```python
from build123d import *

# Parameters (mm, degrees)
SKETCH1_W           = 98
SKETCH1_H           = 55
BOSS_EXTRUDE1_DEPTH = 2
SKETCH2_W           = 98
SKETCH2_H           = 55
SKETCH2_W_2         = 95
SKETCH2_H_2         = 52
BOSS_EXTRUDE2_DEPTH = 9
SKETCH3_R           = 4
SKETCH3_R_2         = 1.8
BOSS_EXTRUDE3_DEPTH = 7


with BuildPart() as part:
    # Sketch1 → Boss-Extrude1 (new body)
    with BuildSketch(Plane.XY):
        with Locations((49, -27.5)):
            Rectangle(SKETCH1_W, SKETCH1_H)
    extrude(amount=BOSS_EXTRUDE1_DEPTH)

    # Sketch2 → Boss-Extrude2 (add)
    with BuildSketch(Plane.XY.offset(2)):
        with Locations((49, -27.5)):
            Rectangle(SKETCH2_W, SKETCH2_H)
        with Locations((49, -27.5)):
            Rectangle(SKETCH2_W_2, SKETCH2_H_2, mode=Mode.SUBTRACT)
    extrude(amount=BOSS_EXTRUDE2_DEPTH)

    # Sketch3 → Boss-Extrude3 (add)
    with BuildSketch(Plane.XY.offset(2)):
        with Locations((89.5, -8.5)):
            Circle(SKETCH3_R)
        with Locations((89.5, -8.5)):
            Circle(SKETCH3_R_2, mode=Mode.SUBTRACT)
        with Locations((89.5, -48.5)):
            Circle(SKETCH3_R)
        with Locations((89.5, -48.5)):
            Circle(SKETCH3_R_2, mode=Mode.SUBTRACT)
        with Locations((6.5, -48.5)):
            Circle(SKETCH3_R)
        with Locations((6.5, -48.5)):
            Circle(SKETCH3_R_2, mode=Mode.SUBTRACT)
        with Locations((23.5, -8.5)):
            Circle(SKETCH3_R)
        with Locations((23.5, -8.5)):
            Circle(SKETCH3_R_2, mode=Mode.SUBTRACT)
    extrude(amount=BOSS_EXTRUDE3_DEPTH)


solid = part.part
```
Input: part model. Units: mm. Frame: model coordinates. A direction names the side the tool comes from. Round coordinates to 2 decimals unless told otherwise and drop trailing zeros. Loops run counter-clockwise (first coordinate to the right, second up) from the corner with the lowest first, then second, coordinate; pieces in that order, holes last. Notation, with made-up numbers: M 3,-35 L 40,-35 A16 ccw 40,-15 Z; hole C 34,29 d9. An arc over 180 degrees is marked long. Answer in a Markdown table with one row per item. Add a question column.
1. Section D-D (x = 45.5). Output: boundary loops of the cut face in (y, z), and give its area (3 significant figures).
2. Section C-C (y = -8.5). Output: boundary loops of the cut face in (x, z), and give its area (3 significant figures).
3. Mould query, pull axis Y, two halves, no side actions, for faces 3 (the face through (6.266, -46.715, 5.451)), 4 (the face through (48, 0, 5)), 5 (the face through (20.3, -10.9, 5.5)), 6 (the face through (98, -28, 5)). Classes: released by +Y, released by -Y, zero draft, split by the parting line, or undercut.
4. Contact query for flat-ended pins moving along their axis: pin 1 (5 mm diameter, centred on x = 39.5, y = -44, fed in from -Z); pin 2 (6.5 mm diameter, centred on x = 24, y = -10.5, fed in from +Z); pin 3 (1.1 mm diameter, centred on x = 6.5, y = -47.5, fed in from +Z). Output: stop coordinate, or through.
5. Ray query, probe 1 along Y at (x, z) = (6.5, 6.5); probe 2 along Y at (x, z) = (23.5, 7.5); probe 3 along Y at (x, z) = (89.5, 6). Return the intervals inside material, ascending.
6. Section B-B (x = 6.5). Output: boundary loops of the cut face in (y, z).
7. Set-up query: faces 1 (the face through (96.5, -28, 6)), 2 (the face through (48, -27, 0)). Return all of +Z, -Z, +X, -X, +Y, -Y with unobstructed straight access to the full face (end or side cutting, diameter ignored); none if empty.
8. Section A-A (z = 7.5). Give the number of separate pieces and of enclosed holes in the cut face, and give its area (3 significant figures).
Values follow:
| question | item | result |
|---|---|---|
| 1 | outline | M -55,0 L 0,0 L 0,11 L -1.5,11 L -1.5,2 L -53.5,2 L -53.5,11 L -55,11 Z |
| 1 | area | 137 mm^2 |
| 2 | outline | M 0,0 L 98,0 L 98,11 L 96.5,11 L 96.5,2 L 93.5,2 L 93.5,9 L 91.3,9 L 91.3,2 L 87.7,2 L 87.7,9 L 85.5,9 L 85.5,2 L 27.5,2 L 27.5,9 L 25.3,9 L 25.3,2 L 21.7,2 L 21.7,9 L 19.5,9 L 19.5,2 L 1.5,2 L 1.5,11 L 0,11 Z |
| 2 | area | 285 mm^2 |
| 3 | face 3 | undercut |
| 3 | face 4 | released by +Y |
| 3 | face 5 | undercut |
| 3 | face 6 | zero draft |
| 4 | pin 1 | z = 0 |
| 4 | pin 2 | z = 9 |
| 4 | pin 3 | z = 2 |
| 5 | probe 1 | -55 to -53.5, -52.5 to -50.3, -46.7 to -44.5, -1.5 to 0 |
| 5 | probe 2 | -55 to -53.5, -12.5 to -10.3, -6.7 to -4.5, -1.5 to 0 |
| 5 | probe 3 | -55 to -53.5, -52.5 to -50.3, -46.7 to -44.5, -12.5 to -10.3, -6.7 to -4.5, -1.5 to 0 |
| 6 | outline | M -55,0 L 0,0 L 0,11 L -1.5,11 L -1.5,2 L -44.5,2 L -44.5,9 L -46.7,9 L -46.7,2 L -50.3,2 L -50.3,9 L -52.5,9 L -52.5,2 L -53.5,2 L -53.5,11 L -55,11 Z |
| 7 | face 1 | +Z |
| 7 | face 2 | -Z, +X, -X, +Y, -Y |
| 8 | separate pieces | 5 |
| 8 | enclosed holes | 5 |
| 8 | area | 610 mm^2 |
